```python
from build123d import *

# Parameters (mm, degrees)
F0_R     = 57.15
F0_R_2   = 4.699
F0_R_3   = 1.524
F1_DEPTH = 25.4


with BuildPart() as f1:
    # F0 (on Top) → F1 (new body)
    with BuildSketch(Plane.XY):
        Circle(F0_R)
        with Locations((-0.012471, -45.568732)):
            Circle(F0_R_2, mode=Mode.SUBTRACT)
        with Locations((-22.799638, -39.458828)):
            Circle(F0_R_2, mode=Mode.SUBTRACT)
        with Locations((-39.478951, -22.773912)):
            Circle(F0_R_2, mode=Mode.SUBTRACT)
        with BuildLine():
            Line((-9.164514, -5.567105), (-18.896484, -20.143289))
            Line((-18.896484, -20.143289), (-22.883833, -21.164274))
            Line((-22.883833, -21.164274), (-29.347375, -22.819305))
            Line((-29.347375, -22.819305), (-30.972017, -23.235305))
            ThreePointArc((-30.972017, -23.235305), (-31.659849, -19.410562), (-33.976573, -16.290536))
            Line((-33.976573, -16.290536), (-33.618292, -15.868193))
            Line((-33.618292, -15.868193), (-29.22395, -10.68813))
            Line((-29.22395, -10.68813), (-26.096301, -7.001249))
            Line((-26.096301, -7.001249), (-9.164514, -5.567105))
        make_face(mode=Mode.SUBTRACT)
        with BuildLine():
            Line((-17.009683, -22.806496), (-5.869526, -6.121182))
            ThreePointArc((-5.869526, -6.121182), (-4.06054, -7.445281), (-1.967811, -8.249117))
            Line((-1.967811, -8.249117), (-10.278486, -25.94343))
            Line((-10.278486, -25.94343), (-8.225538, -31.679786))
            ThreePointArc((-8.225538, -31.679786), (-15.640641, -28.751325), (-22.127766, -24.117013))
            Line((-22.127766, -24.117013), (-17.009683, -22.806496))
        make_face(mode=Mode.SUBTRACT)
        with BuildLine():
            Line((-28.255846, 3.327569), (-8.235862, 2.022568))
            ThreePointArc((-8.235862, 2.022568), (-8.478073, -0.20611), (-8.12785, -2.420384))
            Line((-8.12785, -2.420384), (-27.606912, -4.070285))
            Line((-27.606912, -4.070285), (-31.548269, -8.716368))
            ThreePointArc((-31.548269, -8.716368), (-32.719698, -0.83047), (-31.949829, 7.104701))
            Line((-31.949829, 7.104701), (-28.255846, 3.327569))
        make_face(mode=Mode.SUBTRACT)
        with Locations((22.776746, -39.46648)):
            Circle(F0_R_2, mode=Mode.SUBTRACT)
        with BuildLine():
            Line((0.238997, -10.720255), (7.996358, -26.43648))
            Line((7.996358, -26.43648), (6.886883, -30.400118))
            Line((6.886883, -30.400118), (5.08841, -36.825225))
            Line((5.08841, -36.825225), (4.636356, -38.440205))
            ThreePointArc((4.636356, -38.440205), (0.980115, -37.123514), (-2.880269, -37.569844))
            Line((-2.880269, -37.569844), (-3.066888, -37.048391))
            Line((-3.066888, -37.048391), (-5.355783, -30.652748))
            Line((-5.355783, -30.652748), (-6.984892, -26.100684))
            Line((-6.984892, -26.100684), (0.238997, -10.720255))
        make_face(mode=Mode.SUBTRACT)
        with BuildLine():
            Line((11.246163, -26.134065), (2.366336, -8.143749))
            ThreePointArc((2.366336, -8.143749), (4.417533, -7.239172), (6.160039, -5.828732))
            Line((6.160039, -5.828732), (17.328426, -21.873144))
            Line((17.328426, -21.873144), (23.32273, -22.963418))
            ThreePointArc((23.32273, -22.963418), (17.079057, -27.920855), (9.822063, -31.221714))
            Line((9.822063, -31.221714), (11.246163, -26.134065))
        make_face(mode=Mode.SUBTRACT)
        with BuildLine():
            Line((9.403511, -5.15315), (26.892842, -6.293191))
            Line((26.892842, -6.293191), (29.770716, -9.235843))
            Line((29.770716, -9.235843), (34.435785, -14.00592))
            Line((34.435785, -14.00592), (35.608372, -15.204901))
            ThreePointArc((35.608372, -15.204901), (32.639964, -17.712953), (31.096305, -21.279308))
            Line((31.096305, -21.279308), (30.551404, -21.180199))
            Line((30.551404, -21.180199), (23.868167, -19.964618))
            Line((23.868167, -19.964618), (19.11141, -19.099436))
            Line((19.11141, -19.099436), (9.403511, -5.15315))
        make_face(mode=Mode.SUBTRACT)
        with Locations((39.461662, -22.787167)):
            Circle(F0_R_2, mode=Mode.SUBTRACT)
        with Locations((-45.581203, 0.015305)):
            Circle(F0_R_2, mode=Mode.SUBTRACT)
        with Locations((-39.471299, 22.802472)):
            Circle(F0_R_2, mode=Mode.SUBTRACT)
        with BuildLine():
            Line((-9.403511, 5.15315), (-26.892842, 6.293191))
            Line((-26.892842, 6.293191), (-29.770716, 9.235843))
            Line((-29.770716, 9.235843), (-34.435785, 14.00592))
            Line((-34.435785, 14.00592), (-35.608372, 15.204901))
            ThreePointArc((-35.608372, 15.204901), (-32.639964, 17.712953), (-31.096305, 21.279308))
            Line((-31.096305, 21.279308), (-30.551404, 21.180199))
            Line((-30.551404, 21.180199), (-23.868167, 19.964618))
            Line((-23.868167, 19.964618), (-19.11141, 19.099436))
            Line((-19.11141, 19.099436), (-9.403511, 5.15315))
        make_face(mode=Mode.SUBTRACT)
        with BuildLine():
            Line((-11.246163, 26.134065), (-2.366336, 8.143749))
            ThreePointArc((-2.366336, 8.143749), (-4.417533, 7.239172), (-6.160039, 5.828732))
            Line((-6.160039, 5.828732), (-17.328426, 21.873144))
            Line((-17.328426, 21.873144), (-23.32273, 22.963418))
            ThreePointArc((-23.32273, 22.963418), (-17.079057, 27.920855), (-9.822063, 31.221714))
            Line((-9.822063, 31.221714), (-11.246163, 26.134065))
        make_face(mode=Mode.SUBTRACT)
        with BuildLine():
            Line((-0.238997, 10.720255), (-7.996358, 26.43648))
            Line((-7.996358, 26.43648), (-6.886883, 30.400118))
            Line((-6.886883, 30.400118), (-5.08841, 36.825225))
            Line((-5.08841, 36.825225), (-4.636356, 38.440205))
            ThreePointArc((-4.636356, 38.440205), (-0.980115, 37.123514), (2.880269, 37.569844))
            Line((2.880269, 37.569844), (3.066888, 37.048391))
            Line((3.066888, 37.048391), (5.355783, 30.652748))
            Line((5.355783, 30.652748), (6.984892, 26.100684))
            Line((6.984892, 26.100684), (-0.238997, 10.720255))
        make_face(mode=Mode.SUBTRACT)
        with Locations((-22.786383, 39.481785)):
            Circle(F0_R_2, mode=Mode.SUBTRACT)
        Circle(F0_R_3, mode=Mode.SUBTRACT)
        with BuildLine():
            Line((28.255846, -3.327569), (8.235862, -2.022568))
            ThreePointArc((8.235862, -2.022568), (8.478073, 0.20611), (8.12785, 2.420384))
            Line((8.12785, 2.420384), (27.606912, 4.070285))
            Line((27.606912, 4.070285), (31.548269, 8.716368))
            ThreePointArc((31.548269, 8.716368), (32.719698, 0.83047), (31.949829, -7.104701))
            Line((31.949829, -7.104701), (28.255846, -3.327569))
        make_face(mode=Mode.SUBTRACT)
        with BuildLine():
            Line((17.009683, 22.806496), (5.869526, 6.121182))
            ThreePointArc((5.869526, 6.121182), (4.06054, 7.445281), (1.967811, 8.249117))
            Line((1.967811, 8.249117), (10.278486, 25.94343))
            Line((10.278486, 25.94343), (8.225538, 31.679786))
            ThreePointArc((8.225538, 31.679786), (15.640641, 28.751325), (22.127766, 24.117013))
            Line((22.127766, 24.117013), (17.009683, 22.806496))
        make_face(mode=Mode.SUBTRACT)
        with BuildLine():
            Line((9.164514, 5.567105), (18.896484, 20.143289))
            Line((18.896484, 20.143289), (22.883833, 21.164274))
            Line((22.883833, 21.164274), (29.347375, 22.819305))
            Line((29.347375, 22.819305), (30.972017, 23.235305))
            ThreePointArc((30.972017, 23.235305), (31.659849, 19.410562), (33.976573, 16.290536))
            Line((33.976573, 16.290536), (33.618292, 15.868193))
            Line((33.618292, 15.868193), (29.22395, 10.68813))
            Line((29.22395, 10.68813), (26.096301, 7.001249))
            Line((26.096301, 7.001249), (9.164514, 5.567105))
        make_face(mode=Mode.SUBTRACT)
        with Locations((45.571566, 0)):
            Circle(F0_R_2, mode=Mode.SUBTRACT)
        with Locations((39.469314, 22.789217)):
            Circle(F0_R_2, mode=Mode.SUBTRACT)
        with Locations((22.790001, 39.474133)):
            Circle(F0_R_2, mode=Mode.SUBTRACT)
        with Locations((0.002834, 45.584037)):
            Circle(F0_R_2, mode=Mode.SUBTRACT)
    extrude(amount=F1_DEPTH)


solid = f1.part
```
Verification items for the finished model (mm, model axes). Give positions to 0.01 mm unless a question says otherwise; leave off trailing zeros. Loops run counter-clockwise (first coordinate to the right, second up) from the corner with the lowest first, then second, coordinate; pieces in that order, holes last. Notation, with made-up numbers: M 89,17 L 139,17 A24 ccw 139,44 Z; hole C 39.25,56.25 d5. An arc over 180 degrees is marked long. Return JSON: item names as keys, results as strings.
1) Gauge pin test, flat ends, axial feed: P1, Ø11, axis at x = -22.79, y = 39.48, coming from the +Z side; P2, Ø1.5, axis at y = -13, z = 13.5, coming from the +X side; P3, Ø5.5, axis at x = -39.48, y = -22.77, coming from the -Z side; P4, Ø12, axis at y = -40, z = 12.5, coming from the +X side. Record the tip position at first contact, or that the pin passes through.
Findings:
{"P1": "stops at z = 25.4", "P2": "stops at x = 55.82", "P3": "passes through", "P4": "stops at x = 45.94"}
2) Mould release check, pull along Y, two halves, no side actions. Record for faces 1 (the cylindrical face through (-17.174, 27.862, 12.522)), 2 (the flat face through (-1, -12, 0)): released by +Y, released by -Y, zero draft, split by the parting line, or undercut.
Findings:
{"face 1": "undercut", "face 2": "zero draft"}
3) Material ranges on L1, parallel to X at y = -36, z = 1.75; L2, parallel to X at y = 12.5, z = 23.25; L3, parallel to X at y = 15.5, z = 9.75, recorded low to high. Write a range as [from, to].
Findings:
{"L1": "x = [-44.39, -25.98], [-19.62, -3.44], [5.32, 19.6], [25.95, 44.39]", "L2": "x = [-55.77, -32.96], [-14.52, -10.8], [-4.52, -1.12], [0.6, 3.96], [10.13, 13.79], [30.76, 55.77]", "L3": "x = [-55.01, -35.08], [-16.61, -12.89], [-6, -2.6], [2.01, 5.37], [12.13, 15.8], [33.31, 55.01]"}
4) Section check B-B, the plane z = 11.25. Count the separate pieces of the cut face and the enclosed holes in it, and give its area (3 significant figures).
Findings:
{"separate pieces": "1", "enclosed holes": "25", "area": "6,930 mm2"}
5) Section check A-A, the plane x = -14. Enter the section's corners in (y, z), and give its area (3 significant figures).
Findings:
{"outline": "M -55.41,0 L -29.58,0 L -29.58,25.4 L -55.41,25.4 Z; M -18.3,0 L -12.81,0 L -12.81,25.4 L -18.3,25.4 Z; M -5.98,0 L -2.92,0 L -2.92,25.4 L -5.98,25.4 Z; M 2.4,0 L 5.45,0 L 5.45,25.4 L 2.4,25.4 Z; M 11.76,0 L 17.09,0 L 17.09,25.4 L 11.76,25.4 Z; M 29.58,0 L 55.41,0 L 55.41,25.4 L 29.58,25.4 Z", "area": "1,740 mm2"}
